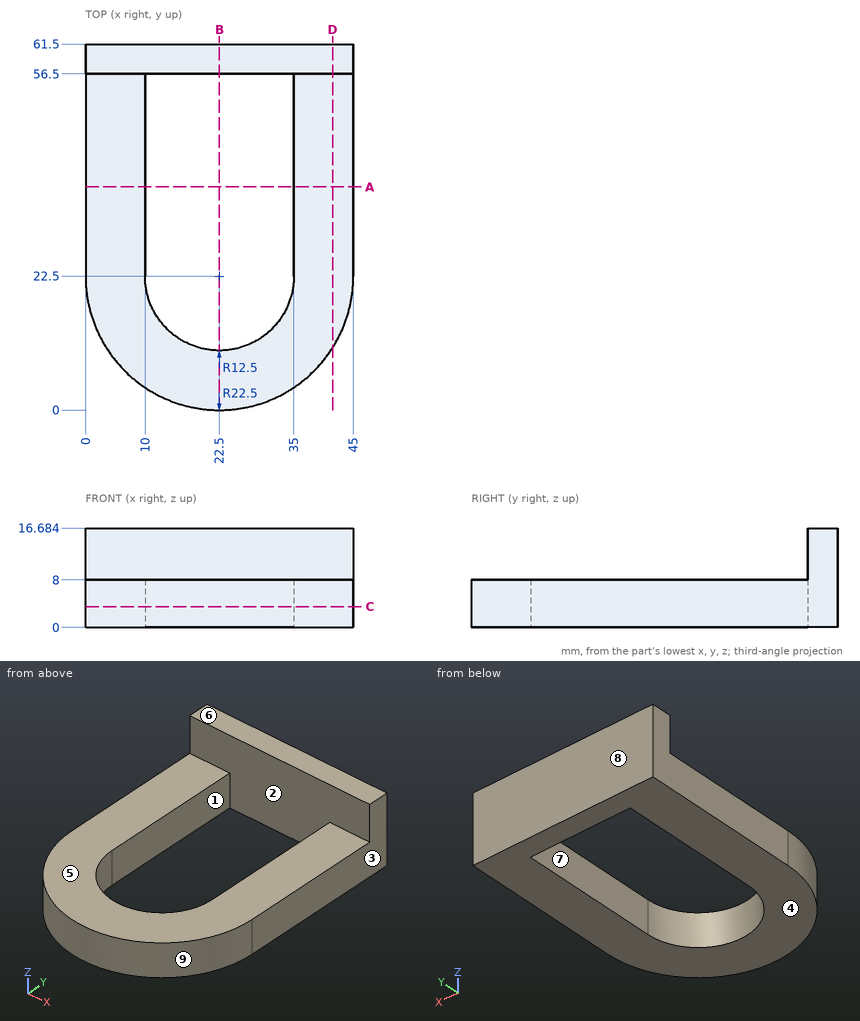
Print and shaded views of the part. All mm, measured from the part's lowest x, y and z. A direction names the side the tool comes from. Coordinates: 2 decimals unless noted, no trailing zeros. Order: outer loops, then holes, each group sorted by start corner. A loop starts at its lowest first (then second) coordinate and runs counter-clockwise, first axis right, second up. Notation, with made-up numbers: M 44,63.25 L 98,63.25 A33 cw 98,100.25 Z; hole C -21.5,52.5 d8. An arc over 180 degrees is marked long. Write each question's results on one line, items separated by ' | '. Start each with the question number.
Q1. Cut at D-D (x = 41.5). List the corners of the cut face in (y, z).
Q2. Which spindle directions (+Z, -Z, +X, -X, +Y, -Y) get a long thin tool onto all of the face, cutting with end or side? Do the marked faces 1, 2, 3, 4 and 5. Say none if no direction does.
Q3. Cut at C-C (z = 3.5). List the corners of the cut face in (x, y).
Q4. Flat gauge pins, fed straight in: P1, Ø22.5, axis at x = 28, y = 39.5, coming from the +Z side; P2, Ø6, axis at x = 5.5, z = 5.5, coming from the -Y side; P3, Ø10, axis at y = 27.5, z = 6.5, coming from the -X side; P4, Ø3, axis at y = 16, z = 3.5, coming from the +X side. Where does each tip first touch, or does it go through?
Q5. Pull direction Y, two halves, no side cores. Call the marked faces 6, 7, 8 and 9: +Y half, -Y half, draft (parallel to the pull), parting line (faces both ways), or undercut.
Q6. Cut at B-B (x = 22.5). List the corners of the cut face in (y, z).
Q7. Drill centre lines: probe 1 along Y at (x, z) = (22, 4.25); probe 2 along Z at (x, y) = (8, 48.5); probe 3 along X at (y, z) = (34, 6.5). Where is each one in solid material? Low to high. Write a range as from..to.
Q8. Cut at A-A (y = 37.5). List the corners of the cut face in (x, z).
Found:
1) outline: M 10.45,0 L 61.5,0 L 61.5,16.68 L 56.5,16.68 L 56.5,8 L 10.45,8 Z
2) face 1: +Z, -Z | face 2: +Z | face 3: +Z, -Z, +X, +Y, -Y | face 4: -Z, +X, -X, +Y, -Y | face 5: +Z, +X, -X, -Y
3) outline: M 0,22.5 A22.5 ccw 45,22.5 L 45,61.5 L 0,61.5 Z; hole M 10,22.5 A12.5 ccw 35,22.5 L 35,56.5 L 10,56.5 Z
4) P1: z = 8 | P2: y = 4.89 | P3: x = 0 | P4: x = 44.44
5) face 6: draft | face 7: undercut | face 8: +Y half | face 9: -Y half
6) outline: M 0,0 L 10,0 L 10,8 L 0,8 Z; M 56.5,0 L 61.5,0 L 61.5,16.68 L 56.5,16.68 Z
7) probe 1: 0.01..10.01, 56.5..61.5 | probe 2: 0..8 | probe 3: 0..10, 35..45
8) outline: M 0,0 L 10,0 L 10,8 L 0,8 Z; M 35,0 L 45,0 L 45,8 L 35,8 Z
